Check sheet for the modelled part. Datum: model origin and axes. Units: mm. Face numbers are marked on the shaded views. A direction names the side the tool comes from. Coordinates: 2 decimals unless noted, no trailing zeros. Order: outer loops, then holes, each group sorted by start corner. A loop starts at its lowest first (then second) coordinate and runs counter-clockwise, first axis right, second up.
1. Cross-section at C-C (z = -0.2). Enter the section's corners in (x, y).
2. Gauge pin test, flat ends, axial feed: pin 1 Ø0.8 at (x, y) = (-0.5, 1.5) entering from +Z; pin 2 Ø1 at (x, z) = (5, -1.5) entering from -Y; pin 3 Ø0.8 at (x, y) = (-0.5, 2) entering from -Z. Record the tip position at first contact, or that the pin passes through.
3. Cross-section at D-D (y = 2.7). Enter the section's corners in (x, z).
4. Thickness scan on line 1 (Y direction, x = 5.5, z = -1.25); line 2 (Y direction, x = 6.25, z = -1.3). Record the ranges inside material, lowest first.
5. Cross-section at B-B (x = 9). Enter the section's corners in (y, z).
6. Set-up check for the marked faces 1 and 2: record each of +Z, -Z, +X, -X, +Y, -Y from which the full face is reachable in a straight line by a thin tool's end or side.
7. Cross-section at A-A (y = 1.3). Enter the section's corners in (x, z).
```python
from build123d import *

# Parameters (mm, degrees)
SKETCH2_W           = 14.5
SKETCH2_H           = 2
BOSS_EXTRUDE1_DEPTH = 3
CUT_EXTRUDE2_DEPTH  = 10
SKETCH6_W           = 1
SKETCH6_H           = 2.899999999
BOSS_EXTRUDE3_DEPTH = 1


with BuildPart() as part:
    # Sketch2 → Boss-Extrude1 (new body)
    with BuildSketch(Plane(origin=(0, 0, 0), x_dir=(1, 0, 0), z_dir=(0, 1, 0))):
        with Locations((7.25, 1)):
            Rectangle(SKETCH2_W, SKETCH2_H)
    extrude(amount=BOSS_EXTRUDE1_DEPTH)

    # Sketch5 → Cut-Extrude2 (cut)
    with BuildSketch(Plane.XY):
        Polygon((14.5, 3), (-1.189290811, -0.137858161), (14.5, -0.137858161), align=None)
    extrude(amount=-CUT_EXTRUDE2_DEPTH, mode=Mode.SUBTRACT)

    # Sketch6 → Boss-Extrude3 (add)
    with BuildSketch(Plane.ZY):
        with Locations((-1, 1.550000001)):
            Rectangle(SKETCH6_W, SKETCH6_H)
    extrude(amount=BOSS_EXTRUDE3_DEPTH)


solid = part.part
```
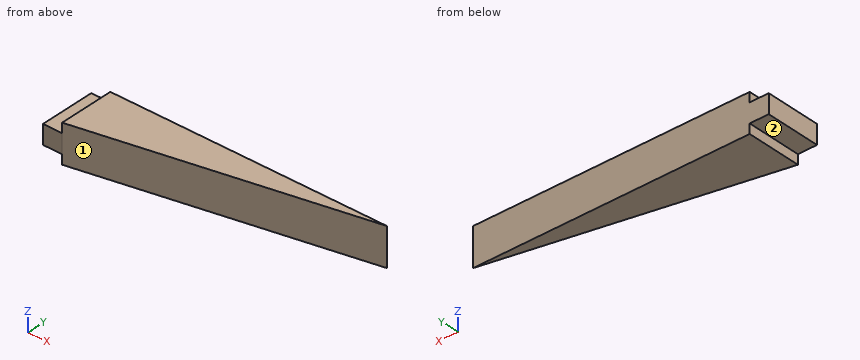
Data:
1. outline: (0, 0.1) - (14.5, 3) - (0, 3) - close
2. pin 1: stops at z = -0.5
2. pin 2: stops at y = 1
2. pin 3: stops at z = -1.5
3. outline: (-1, -1.5) - (0, -1.5) - (0, -2) - (13, -2) - (13, 0) - (0, 0) - (0, -0.5) - (-1, -0.5) - close
4. line 1: y = 1.2 to 3
4. line 2: y = 1.35 to 3
5. outline: (1.9, -2) - (3, -2) - (3, 0) - (1.9, 0) - close
6. face 1: +Z, -Z, +X, -Y
6. face 2: -Z, -X, +Y, -Y
7. outline: (-1, -1.5) - (0, -1.5) - (0, -2) - (6, -2) - (6, 0) - (0, 0) - (0, -0.5) - (-1, -0.5) - close
